Read the model definition and answer for the solid it produces. Units are mm, in the model's axes. Face numbers are marked on the shaded views. Give positions to 0.01 mm unless a question says otherwise; leave off trailing zeros. Loops run counter-clockwise (first coordinate to the right, second up) from the corner with the lowest first, then second, coordinate; pieces in that order, holes last. Notation, with made-up numbers: (43.25, 35) -> (62.25, 35) arc R19 ccw to (62.25, 60) -> close; hole circle Ø4 at (-28.75, 77.5). An arc over 180 degrees is marked (long way). Return JSON: item names as keys, results as strings. Group by question number.
from build123d import *

# Parameters (mm, degrees)
F0_W     = 38.1
F0_H     = 6.35
F0_R     = 2.54
F0_R_2   = 1.1938
F1_DEPTH = 3.175


with BuildPart() as f1:
    # F0 (on Front) → F1 (new body)
    with BuildSketch(Plane.XZ):
        with Locations((19.05, 3.175)):
            Rectangle(F0_W, F0_H)
        with Locations((4.8514, 3.175)):
            Circle(F0_R, mode=Mode.SUBTRACT)
        with Locations((16.51, 3.175)):
            Circle(F0_R_2, mode=Mode.SUBTRACT)
        with Locations((33.02, 3.139029257)):
            Circle(F0_R_2, mode=Mode.SUBTRACT)
    extrude(amount=F1_DEPTH)


solid = f1.part
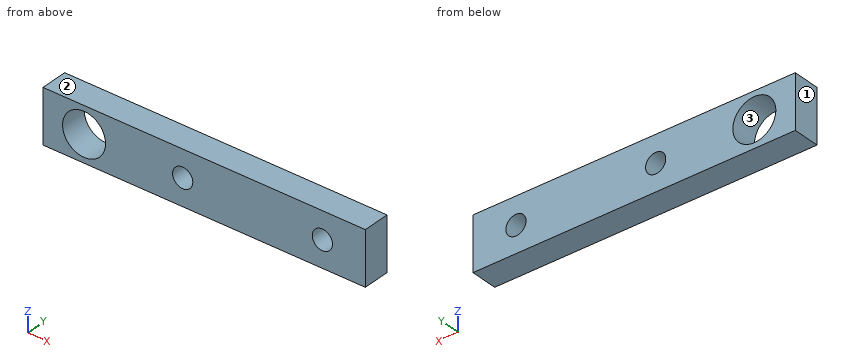
1. Section A-A on x = 16.51 is taken. Determine the outline of the cut face in (y, z) (3 decimals).
2. Straight lines are drawn through the part: line 1 (Z direction, x = 33.02, y = -0.75); line 2 (Z direction, x = 16.51, y = -1.2); line 3 (X direction, y = -1.25, z = 3.75). For each, find the intervals that lie inside material, in ascending order. Write a range as from..to.
3. Determine the mould class of the marked faces 1, 2 and 3 for opening direction Z: pulls with the +Z half, pulls with the -Z half, needs draft (parallel to the pull), parting line crosses it, or undercut.
4. Section C-C on z = 2.5 is taken. Determine the outline of the cut face in (x, y) (3 decimals).
5. Section B-B on z = 1 is taken. Determine the outline of the cut face in (x, y) (3 decimals), then the cut area to 3 significant figures.
6. Section D-D on y = -0.7 is taken. Determine the outline of the cut face in (x, z) (3 decimals), then the cut area to 3 significant figures.
Completed:
{
 "1": {"outline": "(-3.175, 0) -> (0, 0) -> (0, 1.981) -> (-3.175, 1.981) -> close; (-3.175, 4.369) -> (0, 4.369) -> (0, 6.35) -> (-3.175, 6.35) -> close"},
 "2": {"line 1": "z = 0..1.95, 4.33..6.35", "line 2": "z = 0..1.98, 4.37..6.35", "line 3": "x = 0..2.38, 7.33..15.46, 17.56..31.99, 34.05..38.1"},
 "3": {"face 1": "needs draft", "face 2": "pulls with the +Z half", "face 3": "undercut"},
 "4": {"outline": "(0, -3.175) -> (2.403, -3.175) -> (2.403, 0) -> (0, 0) -> close; (7.3, -3.175) -> (15.525, -3.175) -> (15.525, 0) -> (7.3, 0) -> close; (17.495, -3.175) -> (32.012, -3.175) -> (32.012, 0) -> (17.495, 0) -> close; (34.028, -3.175) -> (38.1, -3.175) -> (38.1, 0) -> (34.028, 0) -> close"},
 "5": {"outline": "(0, -3.175) -> (3.54, -3.175) -> (3.54, 0) -> (0, 0) -> close; (6.163, -3.175) -> (38.1, -3.175) -> (38.1, 0) -> (6.163, 0) -> close", "area": "113 mm²"},
 "6": {"outline": "(0, 0) -> (38.1, 0) -> (38.1, 6.35) -> (0, 6.35) -> close; hole circle Ø5.08 at (4.851, 3.175); hole circle Ø2.388 at (16.51, 3.175); hole circle Ø2.388 at (33.02, 3.139)", "area": "213 mm²"}
}
